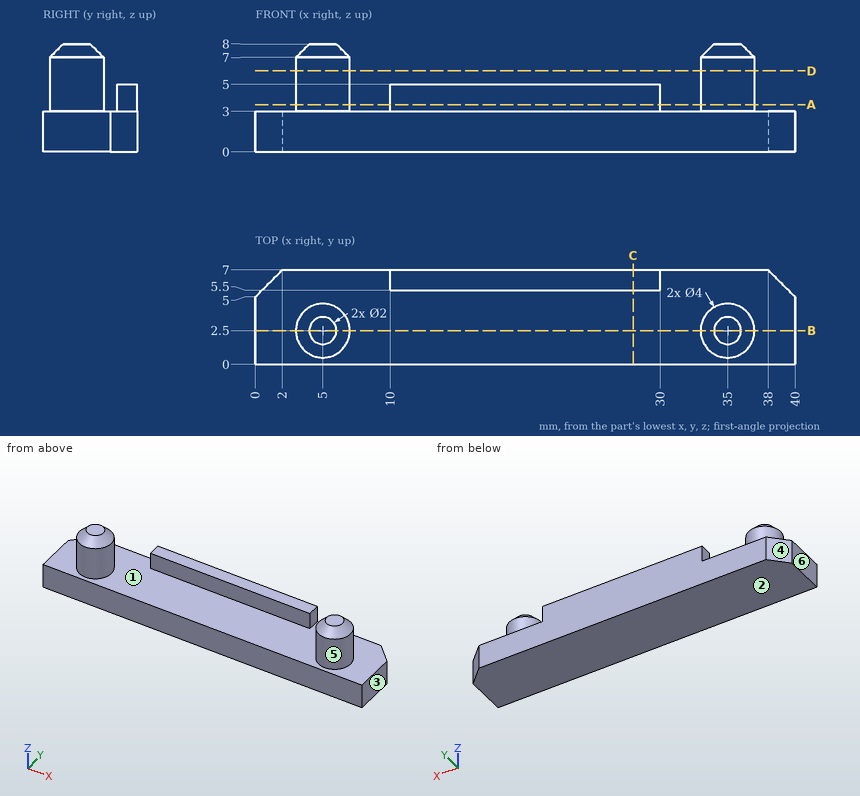
Geometry: see drawing. Coordinates: mm, zero at the bounding-box minimum. A direction names the side the tool comes from. Coordinates: 2 decimals unless noted, no trailing zeros. Loops run counter-clockwise (first coordinate to the right, second up) from the corner with the lowest first, then second, coordinate; pieces in that order, holes last. Notation, with made-up numbers: (8, 37.5) - (39, 37.5) arc R8 ccw to (39, 47.5) - close; hole circle Ø5 at (62, 53). An arc over 180 degrees is marked (long way). Put each result on its own line as item: value. Start each with the question number.
Q1. Cut plane B-B, the plane y = 2.5. Return loops of the section in (x, z), and give its area (3 significant figures).
Q2. Line query: line 1 (X direction, y = 6.75, z = 4.25); line 2 (X direction, y = 4.25, z = 5); line 3 (Z direction, x = 2, y = 4.5). Output: solid intervals per line, ascending.
Q3. Cut plane A-A, the plane z = 3.5. Return loops of the section in (x, y).
Q4. Cut plane D-D, the plane z = 6. Return loops of the section in (x, y).
Q5. Pull-direction query (X, two-part tool) for the marked faces 1, 2, 3 and 4; classes: released by +X, released by -X, zero draft, split by the parting line, or undercut.
Q6. Set-up query: the marked faces 5 and 6. Return all of +Z, -Z, +X, -X, +Y, -Y with unobstructed straight access to the full face (end or side cutting, diameter ignored); none if empty.
Q7. Pin query (flat end, axial travel): pin 1 Ø1 at (x, z) = (24.5, 4.5) entering from -Y; pin 2 Ø4 at (x, z) = (5, 6) entering from -Y; pin 3 Ø3.5 at (x, y) = (22.5, 4) entering from +Z. Return the tip coordinate at first contact, or that it passes through.
Q8. Cut plane C-C, the plane x = 28. Return loops of the section in (y, z), and give its area (3 significant figures).
Filled sheet:
1. outline: (0, 0) - (40, 0) - (40, 3) - (37, 3) - (37, 7) - (36, 8) - (34, 8) - (33, 7) - (33, 3) - (7, 3) - (7, 7) - (6, 8) - (4, 8) - (3, 7) - (3, 3) - (0, 3) - close
1. area: 158 mm²
2. line 1: 10 to 30
2. line 2: 4.03 to 5.97, 34.03 to 35.97
2. line 3: 0 to 3
3. outline: circle Ø4 at (5, 2.5); (10, 5.5) - (30, 5.5) - (30, 7) - (10, 7) - close; circle Ø4 at (35, 2.5)
4. outline: circle Ø4 at (5, 2.5); circle Ø4 at (35, 2.5)
5. face 1: undercut
5. face 2: zero draft
5. face 3: released by +X
5. face 4: released by -X
6. face 5: +Z
6. face 6: +Z, -Z, -X, +Y, -Y
7. pin 1: y = 5.5
7. pin 2: y = 0.5
7. pin 3: z = 5
8. outline: (0, 0) - (7, 0) - (7, 5) - (5.5, 5) - (5.5, 3) - (0, 3) - close
8. area: 24.0 mm²
